```python
from build123d import *

# Parameters (mm, degrees)
F1_DEPTH = 7.86
F3_DEPTH = 25.4
F4_R     = 2.35837
F5_DEPTH = 4
F6_W     = 36.480802
F6_H     = 3.986974
F7_DEPTH = 7


with BuildPart() as f1:
    # F0 (on Front) → F1 (new body)
    with BuildSketch(Plane.XZ):
        Polygon((5.895124, 32.963499), (-8.975978, 32.963499), (-21.356635, -17.178163), (20.118568, -17.178163), align=None)
        Polygon((-8.975978, 32.963499), (-21.356635, 32.963499), (-21.356635, -17.178163), align=None)
        Polygon((20.118568, 32.963499), (5.895124, 32.963499), (20.118568, -17.178163), align=None)
    extrude(amount=F1_DEPTH)

    # F2 (on face) → F3 (cut)
    with BuildSketch(Plane.XZ.offset(7.86)):
        Polygon((-21.356635, 32.963499), (-21.356635, -17.178163), (-11.454494, 32.963499), align=None)
        Polygon((7.754011, 32.963499), (20.118568, -17.178163), (20.118568, 32.963499), align=None)
    extrude(amount=-F3_DEPTH, mode=Mode.SUBTRACT)

    # F4 (on face) → F5 (join)
    with BuildSketch(Plane.XY.offset(32.963499)):
        with Locations((-1.175593, -4.163687)):
            Circle(F4_R)
    extrude(amount=F5_DEPTH)

    # F6 (on face) → F7 (cut)
    with BuildSketch(Plane(origin=(0, 0, -17.178163), x_dir=(1, 0, 0), z_dir=(0, 0, -1))):
        with Locations((-0.981017, 4.267381)):
            Rectangle(F6_W, F6_H)
    extrude(amount=-F7_DEPTH, mode=Mode.SUBTRACT)


solid = f1.part
```
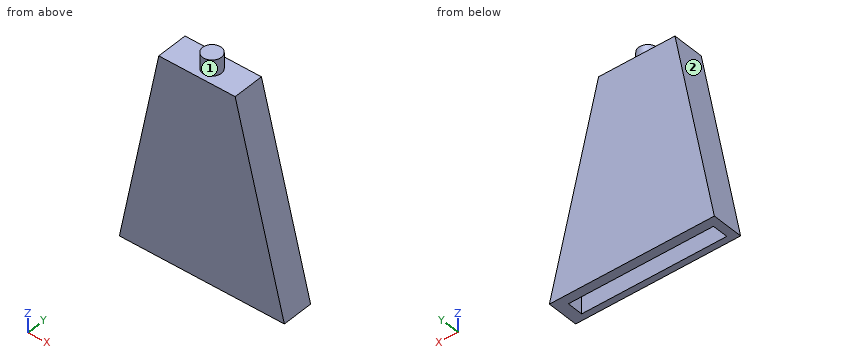
For this review, take the finished solid that the model builds, in its own axes (mm). Face numbers are marked on the shaded views. A direction names the side the tool comes from. Give positions to 0.01 mm unless a question says otherwise; leave off trailing zeros. Write each loop counter-clockwise with the first axis right and the second up, starting at its lowest first coordinate (ties: lowest second). Pieces come first, ordered by that corner, then holes.
Item 1: Wall thickness on probe 1 along Y at (x, z) = (-3, -11); probe 2 along Z at (x, y) = (7, -1.25); probe 3 along Z at (x, y) = (4.5, -3.25): over which ranges is each line inside the solid? List them lowest first.
Item 2: Insertion check: P1, Ø2.5, axis at x = -5.5, y = -3, coming from the +Z side; P2, Ø1.2, axis at y = -3.5, z = -12.5, coming from the +X side; P3, Ø1.5, axis at y = -5, z = 16, coming from the -X side. Each pin has a flat end and moves straight along its axis. Give the tip position at first contact, or say it passes through.
Item 3: Take a section at D-D (x = 16). Give the boundary of the cut face in (y, z).
Item 4: Take a section at B-B (y = -5.25). Give the boundary of the cut face in (x, z), and give its area (3 significant figures).
Item 5: Take a section at A-A (x = -4.5). Give the boundary of the cut face in (y, z), and give its area (3 significant figures).
Item 6: Machinability: for the marked faces 1 and 2, which of the approach directions +Z, -Z, +X, -X, +Y, -Y give a long, thin tool a straight path to every point of the face, cutting with its end or side? Answer none if there is none.
Item 7: Take a section at C-C (z = 1.5). Give the boundary of the cut face in (x, y).
Established:
1. probe 1: y = -7.86 to -6.26, -2.27 to 0
1. probe 2: z = -17.18 to 32.96
1. probe 3: z = -10.18 to 32.96
2. P1: stops at z = 32.96
2. P2: stops at x = 19.11
2. P3: stops at x = -14.95
3. outline: (-7.86, -17.18) - (-6.26, -17.18) - (-6.26, -10.18) - (-2.27, -10.18) - (-2.27, -17.18) - (0, -17.18) - (0, -0.48) - (-7.86, -0.48) - close
4. outline: (-21.36, -17.18) - (-19.22, -17.18) - (-19.22, -10.18) - (17.26, -10.18) - (17.26, -17.18) - (20.12, -17.18) - (7.75, 32.96) - (0.92, 32.96) - (0.92, 36.96) - (-3.27, 36.96) - (-3.27, 32.96) - (-11.45, 32.96) - close
4. area: 1,280 mm2
5. outline: (-7.86, -17.18) - (-6.26, -17.18) - (-6.26, -10.18) - (-2.27, -10.18) - (-2.27, -17.18) - (0, -17.18) - (0, 32.96) - (-7.86, 32.96) - close
5. area: 366 mm2
6. face 1: +Z
6. face 2: +Z, -X, +Y, -Y
7. outline: (-17.67, -7.86) - (15.51, -7.86) - (15.51, 0) - (-17.67, 0) - close
